Job drawing, mm, ordinate dimensions from the low corner. One solid piece. A direction names the side the tool comes from. Give positions to 0.01 mm unless a question says otherwise; leave off trailing zeros. Order: outer loops, then holes, each group sorted by start corner. A loop starts at its lowest first (then second) coordinate and runs counter-clockwise, first axis right, second up.
Item 1: Band-saw the part on B-B on z = 5. Give the cut face in (x, y) (3 decimals).
Item 2: Wall check: L1, parallel to Z at x = 5, y = 3.85 (3 decimals); L2, parallel to Z at x = 5, y = 1.85. Give the ranges that are in metal, low to high.
Item 3: Two-plate mould, pull along X, no slides. Class the marked faces 4, 5 and 6: released by +X, released by -X, zero draft, split by the parting line, or undercut.
Item 4: Band-saw the part on D-D on x = 2.25. Give the cut face in (y, z).
Item 5: Band-saw the part on A-A on x = 5. Give the cut face in (y, z) (3 decimals), plus the area to 3 significant figures.
Item 6: Band-saw the part on C-C on y = 1.45. Give the cut face in (x, z), plus the area to 3 significant figures.
Item 7: Which spindle directions (+Z, -Z, +X, -X, +Y, -Y) get a long thin tool onto all of the face, cutting with end or side? Do the marked faces 1, 2 and 3. Say none if no direction does.
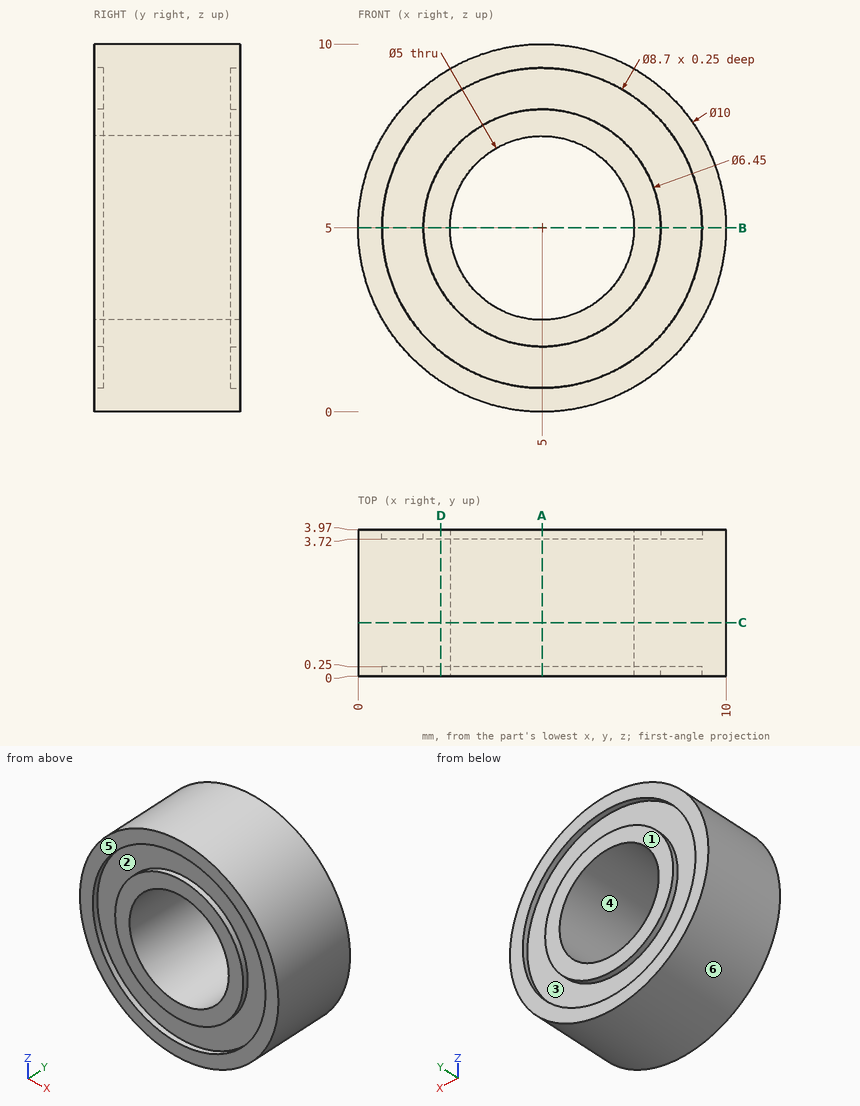
The answers:
1. outline: (0, 0) - (0.65, 0) - (0.65, 0.25) - (1.775, 0.25) - (1.775, 0) - (2.5, 0) - (2.5, 3.97) - (1.775, 3.97) - (1.775, 3.72) - (0.65, 3.72) - (0.65, 3.97) - (0, 3.97) - close; (7.5, 0) - (8.225, 0) - (8.225, 0.25) - (9.35, 0.25) - (9.35, 0) - (10, 0) - (10, 3.97) - (9.35, 3.97) - (9.35, 3.72) - (8.225, 3.72) - (8.225, 3.97) - (7.5, 3.97) - close
2. L1: z = 0 to 0.65, 1.775 to 2.5, 7.5 to 8.225, 9.35 to 10
2. L2: z = 0 to 2.5, 7.5 to 10
3. face 4: undercut
3. face 5: zero draft
3. face 6: split by the parting line
4. outline: (0, 0.82) - (3.97, 0.82) - (3.97, 1.63) - (3.72, 1.63) - (3.72, 3.32) - (3.97, 3.32) - (3.97, 6.68) - (3.72, 6.68) - (3.72, 8.37) - (3.97, 8.37) - (3.97, 9.18) - (0, 9.18) - (0, 8.37) - (0.25, 8.37) - (0.25, 6.68) - (0, 6.68) - (0, 3.32) - (0.25, 3.32) - (0.25, 1.63) - (0, 1.63) - close
5. outline: (0, 0) - (3.97, 0) - (3.97, 0.65) - (3.72, 0.65) - (3.72, 1.775) - (3.97, 1.775) - (3.97, 2.5) - (0, 2.5) - (0, 1.775) - (0.25, 1.775) - (0.25, 0.65) - (0, 0.65) - close; (0, 7.5) - (3.97, 7.5) - (3.97, 8.225) - (3.72, 8.225) - (3.72, 9.35) - (3.97, 9.35) - (3.97, 10) - (0, 10) - (0, 9.35) - (0.25, 9.35) - (0.25, 8.225) - (0, 8.225) - close
5. area: 18.7 mm2
6. outline: circle Ø10 at (5, 5); hole circle Ø5 at (5, 5)
6. area: 58.9 mm2
7. face 1: +Z, -Z, +X, -X, +Y
7. face 2: -Y
7. face 3: +Y
